The listing builds one solid part. Answer for the finished solid, in the listing's coordinates (mm). A direction names the side the tool comes from. Give positions to 0.01 mm unless a question says otherwise; leave off trailing zeros. Write each loop counter-clockwise with the first axis right and the second up, starting at its lowest first coordinate (ties: lowest second). Pieces come first, ordered by that corner, then holes. Notation, with made-up numbers: (-19, 5) -> (1, 5) arc R38 cw to (1, 44) -> close; hole circle Ø1 at (31, 82). An arc over 180 degrees is marked (long way). Put each result on its own line as item: value. Start each with the question number.
1) Flat-ended cylindrical pins translate along their axes: pin 1 Ø3 at (y, z) = (-2.5, 1.5) entering from -X; pin 2 Ø5 at (x, z) = (7, 3.5) entering from -Y; pin 3 Ø5 at (x, z) = (-2, -5) entering from -Y; pin 4 Ø1 at (x, z) = (-1.5, 3.5) entering from +Y. Find the tip coordinate at first contact, or state that the pin passes through.
2) A cutting plane is placed at C-C (x = -8.5). Write down the section's boundary in (y, z).
3) Find the intervals of material crossed by line 1 along X through (y, z) = (2.25, -6.5); line 2 along Z through (x, y) = (-8.5, -0.25); line 3 along Y through (x, z) = (6.25, 0.5), in increasing order. Write a range as from..to.
4) A cutting plane is placed at A-A (z = 0). Write down the section's boundary in (x, y), then the cut area to 3 significant figures.
5) For faces 1 (the flat face through (11.365, 0, 0)), 2 (the cylindrical face through (-1.99, -1.55, 4.91)), determine the directions among +Z, -Z, +X, -X, +Y, -Y from which every point of the face is accessible in a straight line to the end or side of a thin tool.
6) For a pull along X with two mould halves and no side action, classify faces 3 (the cylindrical face through (9.851, -0.33, -7.493)), 4 (the cylindrical face through (7.19, 4.05, -0.9)), 5 (the flat face through (8.365, -4, -4)) as released by +X, released by -X, zero draft, split by the parting line, or undercut.
from build123d import *

# Parameters (mm, degrees)
F2_SIZE = 0.5
F3_SIZE = 3


with BuildPart() as f1:
    # F0 (on Front) → F1 (revolve)
    with BuildSketch(Plane.XZ):
        with BuildLine():
            Line((-12.635403, 5.15), (-12.635403, 0))
            Line((-12.635403, 0), (11.364597, 0))
            Line((11.364597, 0), (11.364597, 7.5))
            Line((11.364597, 7.5), (8.364597, 7.5))
            Line((8.364597, 7.5), (8.364597, 5.15))
            ThreePointArc((8.364597, 5.15), (8.071704, 4.442893), (7.364597, 4.15))
            Line((7.364597, 4.15), (7.019298, 4.15))
            ThreePointArc((7.019298, 4.15), (6.519298, 4.283975), (6.153272, 4.65))
            Line((6.153272, 4.65), (5.864597, 5.15))
            Line((5.864597, 5.15), (-12.635403, 5.15))
        make_face()
    revolve(axis=Axis((-0.635403, 0, 0), (1, 0, 0)))

    # F2
    f2_edges = [f1.edges().sort_by_distance(p)[0] for p in [
        (11.364597, 0, -7.5),
        (8.364597, 0, -7.5),
    ]]
    chamfer(f2_edges, length=F2_SIZE)

    # F3
    f3_edges = [f1.edges().sort_by_distance(p)[0] for p in [
        (-12.635403, 0, -5.15),
    ]]
    chamfer(f3_edges, length=F3_SIZE)


solid = f1.part
Reply:
1. pin 1: stops at x = -12.64
1. pin 2: stops at y = -7.27
1. pin 3: stops at y = -4.5
1. pin 4: stops at y = 4.19
2. outline: circle Ø10.3 at (0, 0)
3. line 1: x = 8.36..11.36
3. line 2: z = -5.14..5.14
3. line 3: y = -4.48..4.48
4. outline: (-12.64, -2.15) -> (-9.64, -5.15) -> (5.86, -5.15) -> (6.15, -4.65) arc R1 cw to (7.02, -4.15) -> (7.36, -4.15) arc R1 cw to (8.36, -5.15) -> (8.36, -7) -> (8.86, -7.5) -> (10.86, -7.5) -> (11.36, -7) -> (11.36, 7) -> (10.86, 7.5) -> (8.86, 7.5) -> (8.36, 7) -> (8.36, 5.15) arc R1 cw to (7.36, 4.15) -> (7.02, 4.15) arc R1 cw to (6.15, 4.65) -> (5.86, 5.15) -> (-9.64, 5.15) -> (-12.64, 2.15) -> close
4. area: 248 mm2
5. face 1: +Z, -Z, +X, +Y, -Y
5. face 2: -X
6. face 3: zero draft
6. face 4: undercut
6. face 5: released by -X
